from build123d import *

# Parameters (mm, degrees)
BOSS_EXTRUDE1_DEPTH      = 75
SKETCH4_R                = 3
CUT_EXTRUDE1_DEPTH       = 3
BOSS_EXTRUDE2_DEPTH      = 4
BOSS_EXTRUDE2_DEPTH_BACK = 3
SKETCH2_R                = 3
SKETCH8_W                = 20.001838136
SKETCH8_H                = 30
BOSS_EXTRUDE6_DEPTH      = 3
SKETCH9_W                = 39.501838136
SKETCH9_H                = 30
BOSS_EXTRUDE7_DEPTH      = 3
SKETCH10_R               = 4.05
BOSS_EXTRUDE8_DEPTH      = 45.001838136
SKETCH11_R               = 4.05
BOSS_EXTRUDE9_DEPTH      = 42
SKETCH12_R               = 11.5
SKETCH12_R_2             = 1.75
CUT_EXTRUDE2_DEPTH       = 42
CUT_EXTRUDE3_START       = -5.5
SKETCH13_R               = 4.05
CUT_EXTRUDE3_DEPTH       = 5.5
SKETCH14_W               = 47.5
SKETCH14_H               = 18.5
BOSS_EXTRUDE11_DEPTH     = 7
CHAMFER1_START           = 96.166522241
CHAMFER1_OUTLINE_W       = 47.5
CHAMFER1_OUTLINE_H       = 10
CHAMFER1_DEPTH           = 4.833477759
SKETCH17_W               = 45
SKETCH17_H               = 18.5
BOSS_EXTRUDE12_DEPTH     = 30
CUT_EXTRUDE5_DEPTH       = 111.611934257
CUT_EXTRUDE5_DEPTH_BACK  = 111.611934257
SKETCH19_R               = 2.75
CUT_EXTRUDE6_DEPTH       = 22
BOSS_EXTRUDE13_START     = -22
SKETCH20_R               = 4.05
BOSS_EXTRUDE13_DEPTH     = 22
SKETCH22_W               = 1
SKETCH22_H               = 10
CUT_EXTRUDE_THIN1_DEPTH  = 51
CHAMFER2_SIZE            = 18.5


with BuildPart() as part:
    # Sketch1 → Boss-Extrude1 (new body)
    with BuildSketch(Plane(origin=(0, 0, 0), x_dir=(1, 0, 0), z_dir=(0, 1, 0))):
        Polygon((0, 0), (0, 40.5), (3, 40.5), (3, -3), (-22, -3), (-22, 0), align=None)
    extrude(amount=BOSS_EXTRUDE1_DEPTH)

    # Sketch4 → Cut-Extrude1 (cut)
    with BuildSketch(Plane(origin=(3, 0, 0), x_dir=(0, 0, -1), z_dir=(1, 0, 0))):
        with Locations((20.25, 27)):
            Circle(SKETCH4_R)
    extrude(amount=-CUT_EXTRUDE1_DEPTH, mode=Mode.SUBTRACT)

    # Sketch2 → Boss-Extrude2 (add, two sides: drawn at the far end of the back side and taken through both)
    with BuildSketch(Plane(origin=(0, 75, 0), x_dir=(1, 0, 0), z_dir=(0, 1, 0)).offset(-BOSS_EXTRUDE2_DEPTH_BACK)):
        Polygon((-0.001838136, 40.5), (-42.001838136, 40.5), (-42.001838136, 0), (-42.001838136, -3), (3, -3), (3, 40.5), align=None)
        with Locations(Location((-19.001838136, 20.25, 0), (0, 0, 270))):
            Circle(SKETCH2_R, mode=Mode.SUBTRACT)
    extrude(amount=BOSS_EXTRUDE2_DEPTH + BOSS_EXTRUDE2_DEPTH_BACK)

    # Sketch8 → Boss-Extrude6 (add)
    with BuildSketch(Plane.XY.offset(3)):
        with Locations((-32.000919068, 57)):
            Rectangle(SKETCH8_W, SKETCH8_H)
    extrude(amount=-BOSS_EXTRUDE6_DEPTH)

    # Sketch9 → Boss-Extrude7 (add)
    with BuildSketch(Plane(origin=(0, 0, -40.5), x_dir=(-1, 0, 0), z_dir=(0, 0, -1))):
        Polygon((42.001838136, 79), (-3, 79), (-3, 0), (0, 0), (0, 72), (42.001838136, 72), align=None)
        with Locations((22.250919068, 57)):
            Rectangle(SKETCH9_W, SKETCH9_H)
    extrude(amount=BOSS_EXTRUDE7_DEPTH)

    # Sketch10 → Boss-Extrude8 (add)
    with BuildSketch(Plane.ZY.offset(42.001838136)):
        Polygon((3, 79), (16.5, 79), (21.5, 74), (21.5, 42), (3, 42), align=None)
        with Locations((11.5, 62)):
            Circle(SKETCH10_R, mode=Mode.SUBTRACT)
    boss_extrude8 = extrude(amount=-BOSS_EXTRUDE8_DEPTH)

    # Sketch11 → Boss-Extrude9 (add)
    with BuildSketch(Plane(origin=(3, 0, 0), x_dir=(0, 0, -1), z_dir=(1, 0, 0))):
        Polygon((-1, 42), (-1, 72), (41.5, 72), (41.5, 42), (43.5, 42), (43.5, 79), (-16.5, 79), (-21.5, 74), (-21.5, 42), (-3, 42), align=None)
        with Locations(Location((-11.5, 62, 0), (0, 0, 180))):
            Circle(SKETCH11_R, mode=Mode.SUBTRACT)
    extrude(amount=BOSS_EXTRUDE9_DEPTH)

    # Mirror3: Boss-Extrude8 across plane
    add(boss_extrude8.mirror(Plane.XY.offset(-20.25)))

    # Sketch12 → Cut-Extrude2 (cut)
    with BuildSketch(Plane.XZ.offset(-72)):
        with Locations(Location((24, -20.25, 0), (0, 0, 270))):
            Circle(SKETCH12_R)
        with Locations(Location((39.317647059, -4.75, 0), (0, 0, 270))):
            Circle(SKETCH12_R_2)
        with Locations(Location((8.317647059, -4.75, 0), (0, 0, 270))):
            Circle(SKETCH12_R_2)
        with Locations(Location((8.317647059, -35.75, 0), (0, 0, 270))):
            Circle(SKETCH12_R_2)
        with Locations(Location((39.317647059, -35.75, 0), (0, 0, 270))):
            Circle(SKETCH12_R_2)
    extrude(amount=-CUT_EXTRUDE2_DEPTH, mode=Mode.SUBTRACT)

    # Sketch13 → Cut-Extrude3 (cut)
    with BuildSketch(Plane(origin=(3, 0, 0), x_dir=(0, 0, -1), z_dir=(1, 0, 0)).offset(CUT_EXTRUDE3_START)):
        Polygon((43.5, 42), (62, 42), (62, 74), (57, 79), (43.5, 79), align=None)
        with Locations(Location((52, 62, 0), (0, 0, 270))):
            Circle(SKETCH13_R, mode=Mode.SUBTRACT)
    extrude(amount=CUT_EXTRUDE3_DEPTH, mode=Mode.SUBTRACT)

    # Sketch14 → Boss-Extrude11 (add)
    with BuildSketch(Plane(origin=(0, 79, 0), x_dir=(1, 0, 0), z_dir=(0, 1, 0))):
        with Locations((21.25, 52.75)):
            Rectangle(SKETCH14_W, SKETCH14_H)
    extrude(amount=-BOSS_EXTRUDE11_DEPTH)

    # Chamfer1: read off the stored shape, not the designer's step
    # Chamfer1 outline → Chamfer1 (cut)
    with BuildSketch(Plane(origin=(0, 0, 0), x_dir=(1, 0, 0), z_dir=(0, 0.7071067811865466, -0.7071067811865486)).offset(CHAMFER1_START)):
        with Locations((21.25, -12)):
            Rectangle(CHAMFER1_OUTLINE_W, CHAMFER1_OUTLINE_H)
    extrude(amount=CHAMFER1_DEPTH, mode=Mode.SUBTRACT)

    # Sketch17 → Boss-Extrude12 (add)
    with BuildSketch(Plane(origin=(0, 72, 0), x_dir=(-1, 0, 0), z_dir=(0, -1, 0))):
        with Locations((-22.5, 52.75)):
            Rectangle(SKETCH17_W, SKETCH17_H)
    extrude(amount=BOSS_EXTRUDE12_DEPTH)

    # Sketch18 → Cut-Extrude5 (cut, two sides: drawn at the far end of the back side and taken through both)
    with BuildSketch(Plane(origin=(0, 0, 1), x_dir=(-1, 0, 0), z_dir=(0, 0, -1)).offset(-CUT_EXTRUDE5_DEPTH_BACK)):
        Polygon((-45, 52), (-45, 42), (-3, 42), align=None)
    extrude(amount=CUT_EXTRUDE5_DEPTH + CUT_EXTRUDE5_DEPTH_BACK, mode=Mode.SUBTRACT)

    # Sketch19 → Cut-Extrude6 (cut)
    with BuildSketch(Plane(origin=(0, 0, 0), x_dir=(-1, 0, 0), z_dir=(0, 0, -1))):
        with Locations((11, 49)):
            Circle(SKETCH19_R)
        with Locations((11, 13.5)):
            Circle(SKETCH19_R)
    extrude(amount=-CUT_EXTRUDE6_DEPTH, mode=Mode.SUBTRACT)

    # Sketch20 → Boss-Extrude13 (add)
    with BuildSketch(Plane(origin=(45, 0, 0), x_dir=(0, 0, -1), z_dir=(1, 0, 0)).offset(BOSS_EXTRUDE13_START)):
        with Locations(Location((-11.5, 62, 0), (0, 0, 180))):
            Circle(SKETCH20_R)
    extrude(amount=BOSS_EXTRUDE13_DEPTH)

    # Sketch22 → Cut-Extrude-Thin1 (cut)
    with BuildSketch(Plane.ZY.offset(42.001838136)):
        with Locations((-52, 57)):
            Rectangle(SKETCH22_W, SKETCH22_H)
        with Locations((11.5, 57)):
            Rectangle(SKETCH22_W, SKETCH22_H)
    extrude(amount=-CUT_EXTRUDE_THIN1_DEPTH, mode=Mode.SUBTRACT)

    # Chamfer2
    chamfer2_edges = [part.edges().sort_by_distance(p)[0] for p in [
        (-9.5, 42, 3),
    ]]
    chamfer(chamfer2_edges, length=CHAMFER2_SIZE - 0.0001)  # a hair under: the kernel refuses the full size


solid = part.part
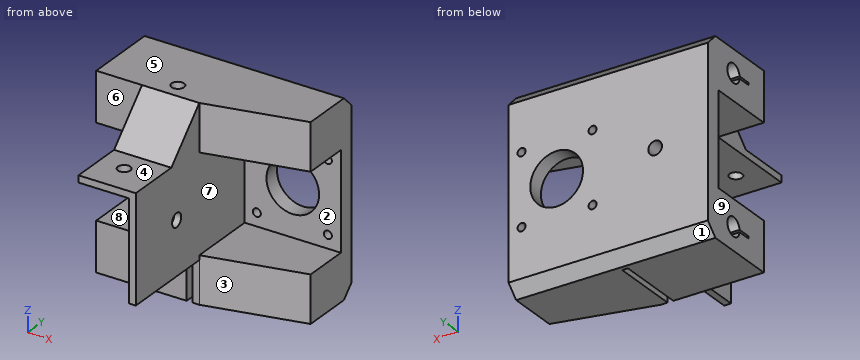
Check sheet for the modelled part. Datum: model origin and axes. Units: mm. Face numbers are marked on the shaded views. A direction names the side the tool comes from. Round coordinates to 2 decimals unless told otherwise and drop trailing zeros. Loops run counter-clockwise (first coordinate to the right, second up) from the corner with the lowest first, then second, coordinate; pieces in that order, holes last. Notation, with made-up numbers: M -34.5,75.25 L 17.5,75.25 A15 cw 17.5,96.25 Z; hole C -3,32.25 d5. An arc over 180 degrees is marked long. One line per question, with ' | ' between items. Start each with the question number.
Item 1: Scan lines: probe 1 along Y at (x, z) = (-11, 1); probe 2 along Z at (x, y) = (-32, 62); probe 3 along X at (y, z) = (67, -58). Record each from-to range of solid material in increasing order.
Item 2: Section check C-C (y = 27). Record the boundary of the cut face in (x, z).
Item 3: Section check A-A (x = -11). State how many separate pieces and enclosed holes the cut face has, and give its area (3 significant figures).
Item 4: Section check D-D (x = 16). Record the boundary of the cut face in (y, z), and give its area (3 significant figures).
Item 5: Release check for a two-part mould opening along Z. For the marked faces 1, 2, 3 and 4 record: released by +Z, released by -Z, zero draft, split by the parting line, or undercut.
Item 6: Set-up check for the marked faces 5, 6, 7, 8 and 9: record each of +Z, -Z, +X, -X, +Y, -Y from which the full face is reachable in a straight line by a thin tool's end or side.
Item 7: Gauge pin test, flat ends, axial feed: pin 1 Ø11 at (x, z) = (-20, -49) entering from -Y; pin 2 Ø2 at (x, y) = (-2.5, 31) entering from -Z; pin 3 Ø10 at (y, z) = (32.5, -42) entering from -X; pin 4 Ø20.5 at (x, z) = (24, -20.25) entering from -Y. Record the tip position at first contact, or that the pin passes through.
Item 8: Section check B-B (z = -35.75). Record the boundary of the cut face in (x, y).
Worked out:
1) probe 1: 0 to 10.75, 16.25 to 46.25, 51.75 to 79 | probe 2: -62 to -56.05, -47.95 to -40.5, 0 to 7.45, 15.55 to 21.5 | probe 3: -42 to -2.5, 0 to 45
2) outline: M -22,0 L 0,0 L 0,-17.25 L 3,-17.25 L 3,6.5 L -22,6.5 Z; M 0,-43.5 L 3,-43.5 L 3,-23.25 L 0,-23.25 Z
3) separate pieces: 3 | enclosed holes: 2 | area: 1,900 mm^2
4) outline: M 45.1,-62 L 74,-62 L 79,-57 L 79,-28.51 L 72,-28.51 L 72,-41.5 L 45.1,-41.5 Z; M 45.1,1 L 72,1 L 72,-11.99 L 79,-11.99 L 79,16.5 L 74,21.5 L 45.1,21.5 Z; hole C 62,11.5 d8.1 | area: 1,500 mm^2
5) face 1: released by -Z | face 2: undercut | face 3: zero draft | face 4: released by +Z
6) face 5: +Z, +X, -X, +Y, -Y | face 6: +Z, -Z, -X, -Y | face 7: +X, -Y | face 8: -X, -Y | face 9: +Z, -Z, -X, +Y, -Y
7) pin 1: y = 42 | pin 2: z = 0 | pin 3: x = 0 | pin 4: through
8) outline: M -42,72 L 0,72 L 0,0 L 3,0 L 3,72 L 6.57,72 L 6.57,79 L -42,79 Z; M 10.07,72 L 37.57,72 L 37.57,79 L 10.07,79 Z; M 41.07,72 L 45,72 L 45,79 L 41.07,79 Z
